The figure shows three views and two pictorial views of one solid part (mm, origin at its lowest corner). Answer the questions. Give positions to 0.01 mm unless a question says otherwise; leave off trailing zeros. Write each loop counter-clockwise with the first axis right and the second up, starting at its lowest first coordinate (ties: lowest second). Pieces come first, ordered by that corner, then holes. Notation, with made-up numbers: (-19.75, 57) -> (22.25, 57) arc R8 ccw to (22.25, 61) -> close; hole circle Ø7 at (-36, 27.5). An arc over 180 degrees is marked (long way). Write each question's results on one line, items separated by ' | '. Start each with the question number.
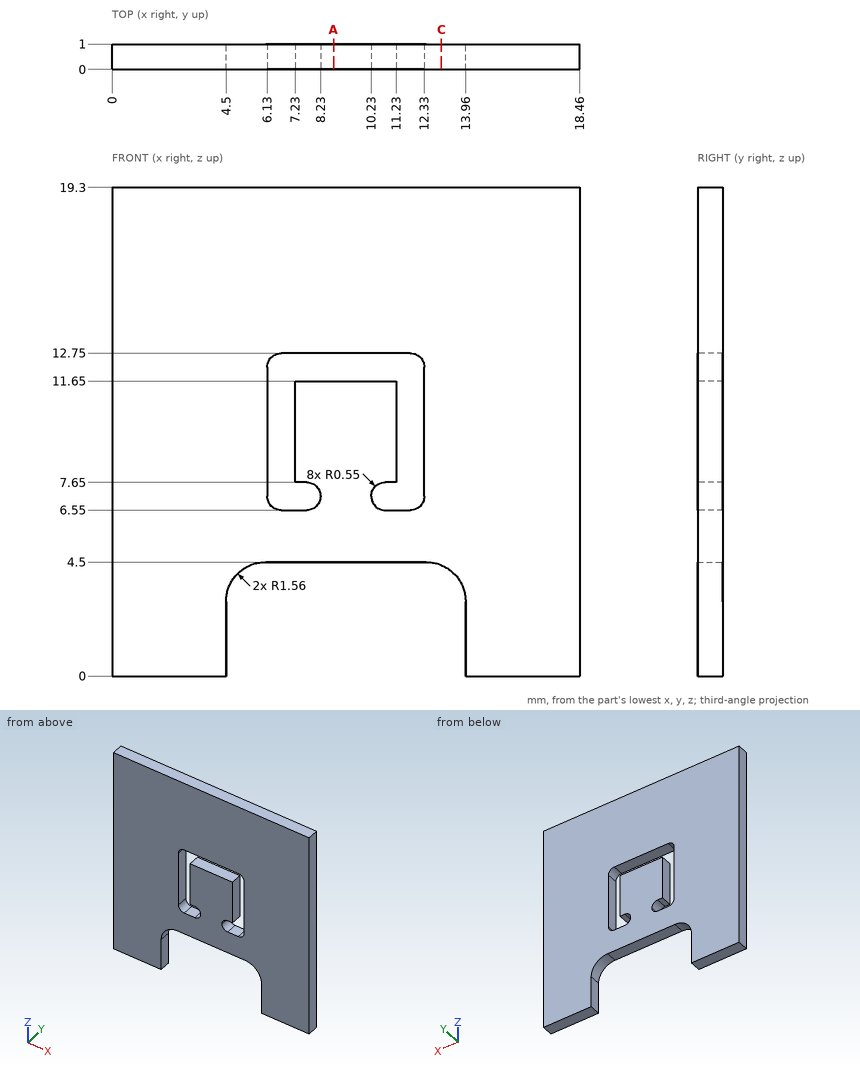
1. Section C-C (x = 13) is taken. Write down the section's boundary in (y, z), then the cut area to 3 significant figures.
2. Section A-A (x = 8.75) is taken. Write down the section's boundary in (y, z), then the cut area to 3 significant figures.
3. Consider probe 1 along Z at (x, y) = (7.5, 0.6); probe 2 along Z at (x, y) = (10, 0.35); probe 3 along Z at (x, y) = (11.75, 0.7). Determine where each line is inside the solid, lowest interval first. Write a range as [from, to].
Results:
1) outline: (0, 4.38) -> (1, 4.38) -> (1, 19.3) -> (0, 19.3) -> close | area: 14.9 mm²
2) outline: (0, 4.5) -> (1, 4.5) -> (1, 11.65) -> (0, 11.65) -> close; (0, 12.75) -> (1, 12.75) -> (1, 19.3) -> (0, 19.3) -> close | area: 13.7 mm²
3) probe 1: z = [4.5, 6.55], [7.65, 11.65], [12.75, 19.3] | probe 2: z = [4.5, 11.65], [12.75, 19.3] | probe 3: z = [4.5, 6.55], [12.75, 19.3]
